from build123d import *

# Parameters (mm, degrees)
F1_DEPTH = 1981.2
F3_DEPTH = 25.4
F4_SIZE  = 5.08


with BuildPart() as f1:
    # F0 (on Right) → F1 (new body)
    with BuildSketch(Plane.YZ):
        with BuildLine():
            Line((-17.145, 0), (0, 0))
            Line((0, 0), (0, 101.6))
            Line((0, 101.6), (-12.7, 101.6))
            Line((-12.7, 101.6), (-12.7, 98.425))
            ThreePointArc((-12.7, 98.425), (-21.680256, 94.705256), (-25.4, 85.725))
            Line((-25.4, 85.725), (-25.4, 38.1))
            Line((-25.4, 38.1), (-17.145, 38.1))
            Line((-17.145, 38.1), (-17.145, 0))
        make_face()
    extrude(amount=F1_DEPTH)

    # F2 (on face) → F3 (cut)
    with BuildSketch(Plane(origin=(0, 0, 0), x_dir=(-1, 0, 0), z_dir=(0, 1, 0))):
        Polygon((-1879.6, 0), (-1981.2, 101.6), (-1981.2, 0), align=None)
        Polygon((0, 0), (0, 101.6), (-101.6, 0), align=None)
    extrude(amount=-F3_DEPTH, mode=Mode.SUBTRACT)

    # F4
    f4_edges = [f1.edges().sort_by_distance(p)[0] for p in [
        (990.6, -25.4, 38.1),
    ]]
    chamfer(f4_edges, length=F4_SIZE)


solid = f1.part
Read the model definition and answer for the solid it produces. Units are mm, in the model's axes. A direction names the side the tool comes from. Round coordinates to 2 decimals unless told otherwise and drop trailing zeros. Write each loop counter-clockwise with the first axis right and the second up, starting at its lowest first coordinate (ties: lowest second). Pieces come first, ordered by that corner, then holes.
1. Straight lines are drawn through the part: L1, parallel to Z at x = 736, y = -15.5; L2, parallel to Y at x = 1273, z = 37.5 (3 decimals); L3, parallel to Z at x = 1267, y = -13.25. For each, find the intervals that lie inside material, in ascending order.
2. The part is cut by section C-C, the plane y = -5. Determine the outline of the cut face in (x, z), then the cut area to 3 significant figures.
3. Which of the six approach directions +Z, -Z, +X, -X, +Y, -Y give full straight-line access (tool end or side, diameter ignored) to faces 1 (the face through (977, -25.4, 65)), 2 (the face through (978, -17.145, 19))?
4. The part is cut by section A-A, the plane x = 265. Determine the outline of the cut face in (y, z) (3 decimals), then the cut area to 3 significant figures.
5. Given pin 1 Ø11.5 at (x, z) = (681, 20.5) entering from -Y (3 decimals); pin 2 Ø12 at (x, y) = (575, -9.5) entering from -Z; pin 3 Ø5 at (x, y) = (640, -19.5) entering from +Z; pin 4 Ø4 at (y, z) = (-15.5, 29.5) entering from +X, each flat-ended and moving along its own axis, determine where each tip first touches the part or whether it passes through.
6. The part is cut by section B-B, the plane z = 63.5. Determine the outline of the cut face in (x, y).
Values:
1. L1: z = 0 to 98.11
1. L2: y = -17.145 to 0
1. L3: z = 0 to 98.41
2. outline: (0, 101.6) - (101.6, 0) - (1879.6, 0) - (1981.2, 101.6) - close
2. area: 191,000 mm2
3. face 1: +Z, -Z, +X, -X, -Y
3. face 2: -Z, +X, -X, -Y
4. outline: (-25.4, 43.18) - (-20.32, 38.1) - (-17.145, 38.1) - (-17.145, 0) - (0, 0) - (0, 101.6) - (-12.7, 101.6) - (-12.7, 98.425) arc R12.7 ccw to (-25.4, 85.725) - close
4. area: 2,180 mm2
5. pin 1: stops at y = -17.145
5. pin 2: stops at z = 0
5. pin 3: stops at z = 97.67
5. pin 4: stops at x = 1911.1
6. outline: (38.1, -25.4) - (1943.1, -25.4) - (1943.1, 0) - (38.1, 0) - close
